Geometry check sheet. Reference: the model listing, model coordinates, mm. Coordinates: 2 decimals unless noted, no trailing zeros. Loops run counter-clockwise (first coordinate to the right, second up) from the corner with the lowest first, then second, coordinate; pieces in that order, holes last. Notation, with made-up numbers: M 52.5,34.25 L 57.5,34.25 A26 cw 57.5,62.25 Z; hole C -5.75,73 d10. An arc over 180 degrees is marked long. Use CSV: the item, a comma, the result in double quotes.
```python
from build123d import *

# Parameters (mm, degrees)
SKETCH1_R               = 4.05
SKETCH1_R_2             = 2.1
BOSS_EXTRUDE1_DEPTH     = 7
SKETCH2_R               = 4.5
SKETCH2_R_2             = 2.1
BOSS_EXTRUDE2_DEPTH     = 9
FILLET1_R               = 0.4
CUT_EXTRUDE1_DEPTH      = 18.219175358
CUT_EXTRUDE1_DEPTH_BACK = 18.219175358
SKETCH3_R               = 0.9
CUT_EXTRUDE2_DEPTH      = 18.219175507
CUT_EXTRUDE2_DEPTH_BACK = 18.219175507
SKETCH4_R               = 0.9
CUT_EXTRUDE3_DEPTH      = 19.631291047
CUT_EXTRUDE3_DEPTH_BACK = 19.631291047
SKETCH6_R               = 0.9
CUT_EXTRUDE4_DEPTH      = 19.631291042
CUT_EXTRUDE4_DEPTH_BACK = 19.631291042
SKETCH7_R               = 0.9
FILLET2_R               = 0.4
FILLET3_R               = 0.4


with BuildPart() as part:
    # Sketch1 → Boss-Extrude1 (new body)
    with BuildSketch(Plane(origin=(0, 0, 0), x_dir=(0, 0, -1), z_dir=(1, 0, 0))):
        Circle(SKETCH1_R)
        Circle(SKETCH1_R_2, mode=Mode.SUBTRACT)
    extrude(amount=BOSS_EXTRUDE1_DEPTH)

    # Sketch2 → Boss-Extrude2 (add)
    with BuildSketch(Plane(origin=(7, 0, 0), x_dir=(0, 0, -1), z_dir=(1, 0, 0))):
        Circle(SKETCH2_R)
        Circle(SKETCH2_R_2, mode=Mode.SUBTRACT)
    extrude(amount=BOSS_EXTRUDE2_DEPTH)

    # Fillet1
    fillet1_edges = [part.edges().sort_by_distance(p)[0] for p in [
        (16, 0, 2.1),
    ]]
    fillet(fillet1_edges, radius=FILLET1_R)

    # Sketch3 → Cut-Extrude1 (cut, two sides: drawn at the far end of the back side and taken through both)
    with BuildSketch(Plane(origin=(0, 0, 0), x_dir=(1, 0, 0), z_dir=(0, 1, 0)).offset(-CUT_EXTRUDE1_DEPTH_BACK)):
        with Locations(Location((12.5, 0, 0), (0, 0, 270))):
            Circle(SKETCH3_R)
    extrude(amount=CUT_EXTRUDE1_DEPTH + CUT_EXTRUDE1_DEPTH_BACK, mode=Mode.SUBTRACT)

    # Sketch4 → Cut-Extrude2 (cut, two sides: drawn at the far end of the back side and taken through both)
    with BuildSketch(Plane.XY.offset(-CUT_EXTRUDE2_DEPTH_BACK)):
        with Locations((14, 0)):
            Circle(SKETCH4_R)
    extrude(amount=CUT_EXTRUDE2_DEPTH + CUT_EXTRUDE2_DEPTH_BACK, mode=Mode.SUBTRACT)

    # Sketch6 → Cut-Extrude3 (cut, two sides: drawn at the far end of the back side and taken through both)
    with BuildSketch(Plane(origin=(0, 2.25, -2.25), x_dir=(1, 0, 0), z_dir=(0, -0.7071067811865488, 0.7071067811865464)).offset(-CUT_EXTRUDE3_DEPTH_BACK)):
        with Locations(Location((11, 0, 0), (0, 0, 270))):
            Circle(SKETCH6_R)
    extrude(amount=CUT_EXTRUDE3_DEPTH + CUT_EXTRUDE3_DEPTH_BACK, mode=Mode.SUBTRACT)

    # Sketch7 → Cut-Extrude4 (cut, two sides: drawn at the far end of the back side and taken through both)
    with BuildSketch(Plane(origin=(0, -2.25, -2.25), x_dir=(1, 0, 0), z_dir=(0, -0.7071067811865438, -0.7071067811865512)).offset(-CUT_EXTRUDE4_DEPTH_BACK)):
        with Locations(Location((9.5, 0, 0), (0, 0, 270))):
            Circle(SKETCH7_R)
    extrude(amount=CUT_EXTRUDE4_DEPTH + CUT_EXTRUDE4_DEPTH_BACK, mode=Mode.SUBTRACT)

    # Fillet2
    fillet2_edges = [part.edges().sort_by_distance(p)[0] for p in [
        (16, 0, 4.5),
    ]]
    fillet(fillet2_edges, radius=FILLET2_R)

    # Fillet3
    fillet3_edges = [part.edges().sort_by_distance(p)[0] for p in [
        (7, 0, 4.5),
    ]]
    fillet(fillet3_edges, radius=FILLET3_R)


solid = part.part
```
1. Section check A-A, the plane y = 0. Record the cut outline in (x, z).
The answers:
outline,"M 0,-4.05 L 7,-4.05 L 7,-4.1 A0.4 ccw 7.4,-4.5 L 13.1,-4.5 L 13.1,-2.1 L 0,-2.1 Z; M 0,2.1 L 13.1,2.1 L 13.1,4.5 L 7.4,4.5 A0.4 ccw 7,4.1 L 7,4.05 L 0,4.05 Z; M 14.9,-4.5 L 15.6,-4.5 A0.4 ccw 16,-4.1 L 16,-2.5 A0.4 ccw 15.6,-2.1 L 14.9,-2.1 Z; M 14.9,2.1 L 15.6,2.1 A0.4 ccw 16,2.5 L 16,4.1 A0.4 ccw 15.6,4.5 L 14.9,4.5 Z"
2. Thickness scan on line 1 (Y direction, x = 8.75, z = 0); line 2 (X direction, y = 2.65, z = 0); line 3 (Z direction, x = 6, y = 1.5). Record the ranges inside material, lowest first. Write a range as [from, to].
The answers:
line 1,"[-4.5, -2.1], [2.1, 4.5]"
line 2,"[0, 11.6], [13.4, 16]"
line 3,"[-3.76, -1.47], [1.47, 3.76]"
3. Section check C-C, the plane x = 14. Record the cut outline in (y, z), plus the area to 3 significant figures.
The answers:
outline,"M -0.9,-4.41 L -0.9,-1.9 A2.1 cw -0.9,1.9 L -0.9,4.41 A4.5 ccw Z; M 0.9,-4.41 A4.5 ccw 0.9,4.41 L 0.9,1.9 A2.1 cw 0.9,-1.9 Z"
area,"41.0 mm^2"
4. Section check D-D, the plane x = 9.25. Record the cut outline in (y, z).
The answers:
outline,"M -3.73,-2.51 L -1.96,-0.74 A2.1 cw 0.74,1.96 L 2.51,3.73 A4.5 ccw Z; M -2.51,-3.73 A4.5 ccw 3.73,2.51 L 1.96,0.74 A2.1 cw -0.74,-1.96 Z"
5. Section check B-B, the plane z = 0. Record the cut outline in (x, y).
The answers:
outline,"M 0,-4.05 L 7,-4.05 L 7,-4.1 A0.4 ccw 7.4,-4.5 L 11.6,-4.5 L 11.6,-2.1 L 0,-2.1 Z; M 0,2.1 L 11.6,2.1 L 11.6,4.5 L 7.4,4.5 A0.4 ccw 7,4.1 L 7,4.05 L 0,4.05 Z; M 13.4,-4.5 L 15.6,-4.5 A0.4 ccw 16,-4.1 L 16,-2.5 A0.4 ccw 15.6,-2.1 L 13.4,-2.1 Z; M 13.4,2.1 L 15.6,2.1 A0.4 ccw 16,2.5 L 16,4.1 A0.4 ccw 15.6,4.5 L 13.4,4.5 Z"
6. Release check for a two-part mould opening along Z. For faces 1 (the flat face through (16, -2, 2)), 2 (the cylindrical face through (3.451, -3.954, 0.878)), 3 (the cylindrical face through (12.77, -3.22, 0.86)) record: +Z half, -Z half, draft (parallel to the pull), parting line (faces both ways), or undercut.
The answers:
face 1,"draft"
face 2,"parting line"
face 3,"undercut"
7. Gauge pin test, flat ends, axial feed: P1, Ø4, axis at x = 4, y = -3.5, coming from the +Z side; P2, Ø4, axis at x = 1.5, z = 2.5, coming from the +Y side; P3, Ø1, axis at x = 7.5, y = 3.5, coming from the -Z side; P4, Ø4, axis at x = 12.5, z = 1.5, coming from the +Y side. Record the tip position at first contact, or that the pin passes through.
The answers:
P1,"z = 3.76"
P2,"y = 4.02"
P3,"z = -3.35"
P4,"y = 4.5"
